```python
from build123d import *

# Parameters (mm, degrees)
SKETCH1_R           = 5.5
BOSS_EXTRUDE1_DEPTH = 2
SKETCH2_R           = 5
BOSS_EXTRUDE2_DEPTH = 8
REVOLVE1_ANGLE      = 180
SKETCH4_W           = 0.5
SKETCH4_H           = 0.5
BOSS_EXTRUDE3_DEPTH = 26


with BuildPart() as part:
    # Sketch1 → Boss-Extrude1 (new body)
    with BuildSketch(Plane(origin=(0, 0, 0), x_dir=(1, 0, 0), z_dir=(0, 1, 0))):
        with Locations(Location((0, 0, 0), (0, 0, 270))):
            Circle(SKETCH1_R)
    extrude(amount=BOSS_EXTRUDE1_DEPTH)

    # Sketch2 → Boss-Extrude2 (add)
    with BuildSketch(Plane(origin=(0, 2, 0), x_dir=(1, 0, 0), z_dir=(0, 1, 0))):
        with Locations(Location((0, 0, 0), (0, 0, 270))):
            Circle(SKETCH2_R)
    extrude(amount=BOSS_EXTRUDE2_DEPTH)

    # Sketch3 → Revolve1 (revolve)
    with BuildSketch(Plane(origin=(0, 10, 0), x_dir=(1, 0, 0), z_dir=(0, 1, 0))):
        with BuildLine():
            Line((0, 5), (0, -5))
            ThreePointArc((0, -5), (5, 0), (0, 5))
        make_face()
    revolve(axis=Axis((0, 10, -5), (0, 0, 1)), revolution_arc=REVOLVE1_ANGLE)

    # Sketch4 → Boss-Extrude3 (add)
    with BuildSketch(Plane.XZ):
        with Locations((-1, 0)):
            Rectangle(SKETCH4_W, SKETCH4_H)
        with Locations((1, 0)):
            Rectangle(SKETCH4_W, SKETCH4_H)
    extrude(amount=BOSS_EXTRUDE3_DEPTH)


solid = part.part
```
The model under review builds one solid part; all positions refer to its coordinate system, in mm. Give positions to 0.01 mm unless a question says otherwise; leave off trailing zeros. Loops run counter-clockwise (first coordinate to the right, second up) from the corner with the lowest first, then second, coordinate; pieces in that order, holes last. Notation, with made-up numbers: (26, -37) -> (48, -37) arc R17 ccw to (48, -12) -> close; hole circle Ø3 at (6.25, 53). An arc over 180 degrees is marked (long way). Use CSV: the item, a comma, the result in double quotes.
1. Consider section B-B, the plane x = 0. Write out the cut boundary in (y, z).
Result:
outline,"(0, -5.5) -> (2, -5.5) -> (2, -5) -> (10, -5) arc R5 ccw to (10, 5) -> (2, 5) -> (2, 5.5) -> (0, 5.5) -> close"
2. Consider section D-D, the plane y = 5. Write out the cut boundary in (x, z), then the cut area to 3 significant figures.
Result:
outline,"circle Ø10 at (0, 0)"
area,"78.5 mm²"
3. Consider section C-C, the plane z = -2.5. Write out the cut boundary in (x, y).
Result:
outline,"(-4.9, 0) -> (4.9, 0) -> (4.9, 2) -> (4.33, 2) -> (4.33, 10) arc R4.33 ccw to (-4.33, 10) -> (-4.33, 2) -> (-4.9, 2) -> close"
4. The part is to be moulded in two halves that separate along X. For faces 1 (the face through (-5.37, 0.99, -1.19)), 2 (the face through (-4.9, 2, 1.6)), say which applies: +X half, -X half, draft (parallel to the pull), parting line (faces both ways), or undercut.
Result:
face 1,"parting line"
face 2,"draft"
5. For P1, Ø5, axis at x = 3, z = 3, coming from the -Y side; P2, Ø0.6, axis at x = -1, y = -11, coming from the +Z side; P3, Ø2, axis at x = 3.5, z = -2, coming from the +Y side, all flat-tipped, find the tip position at first contact; note any pin that passes through.
Result:
P1,"stops at y = 0"
P2,"stops at z = 0.25"
P3,"stops at y = 13.98"
6. To check wall thickness, follow probe 1 along X at (y, z) = (4.5, -0.25); probe 2 along Z at (x, y) = (1, -17.5); probe 3 along Y at (x, z) = (-3.5, -4). State the ranges of each line that lie inside material, in increasing order. Write a range as from..to.
Result:
probe 1,"x = -4.99..4.99"
probe 2,"z = -0.25..0.25"
probe 3,"y = 0..2"
7. Consider section A-A, the plane y = -9.5. Write out the cut boundary in (x, z), then the cut area to 3 significant figures.
Result:
outline,"(-1.25, -0.25) -> (-0.75, -0.25) -> (-0.75, 0.25) -> (-1.25, 0.25) -> close; (0.75, -0.25) -> (1.25, -0.25) -> (1.25, 0.25) -> (0.75, 0.25) -> close"
area,"0.500 mm²"
